Check sheet for the modelled part. Datum: model origin and axes. Units: mm. A direction names the side the tool comes from. Coordinates: 2 decimals unless noted, no trailing zeros. Write each loop counter-clockwise with the first axis right and the second up, starting at its lowest first coordinate (ties: lowest second). Pieces come first, ordered by that corner, then holes. Notation, with made-up numbers: (27, 75.5) -> (67, 75.5) arc R24 cw to (67, 87.5) -> close; hole circle Ø5 at (-37, -32). An arc over 180 degrees is marked (long way). Put each result on its own line as item: value.
```python
from build123d import *

# Parameters (mm, degrees)
SKETCH1_R           = 2.7
SKETCH1_R_2         = 3.55
BOSS_EXTRUDE1_DEPTH = 3.175
CHAMFER1_SIZE       = 3
CUT_EXTRUDE2_REACH  = 5.175
CUT_EXTRUDE3_START  = -3.175
SKETCH8_W           = 11
SKETCH8_H           = 1.8
CUT_EXTRUDE3_DEPTH  = 3.175
SKETCH9_W           = 8.878679656
SKETCH9_H           = 1.6
BOSS_EXTRUDE2_DEPTH = 3.175
BOSS_EXTRUDE3_DEPTH = 3.175
CUT_EXTRUDE4_REACH  = 5.175
CHAMFER3_SIZE       = 1.060660172
CHAMFER4_SIZE       = 3


with BuildPart() as part:
    # Sketch1 → Boss-Extrude1 (new body)
    with BuildSketch(Plane(origin=(0, 0, 0), x_dir=(1, 0, 0), z_dir=(0, 1, 0))):
        Polygon((0, 0), (40, 0), (40, -17.5), (57, -17.5), (57, 37.5), (40, 37.5), (40, 20), (0, 20), align=None)
        with Locations((29, 10)):
            Circle(SKETCH1_R, mode=Mode.SUBTRACT)
        with Locations((9, 10)):
            Circle(SKETCH1_R_2, mode=Mode.SUBTRACT)
        with Locations((48.5, 31.5)):
            Circle(SKETCH1_R, mode=Mode.SUBTRACT)
        with Locations((48.5, -11.5)):
            Circle(SKETCH1_R, mode=Mode.SUBTRACT)
        with Locations((49, 10)):
            Circle(SKETCH1_R, mode=Mode.SUBTRACT)
    extrude(amount=BOSS_EXTRUDE1_DEPTH)

    # Chamfer1
    chamfer1_edges = [part.edges().sort_by_distance(p)[0] for p in [
        (0, 1.5875, -20),
        (40, 1.5875, -37.5),
        (57, 1.5875, -37.5),
        (57, 1.5875, 17.5),
        (40, 1.5875, 17.5),
        (0, 1.5875, 0),
    ]]
    chamfer(chamfer1_edges, length=CHAMFER1_SIZE)

    # Sketch6 → Cut-Extrude2 (cut, up to next)
    with BuildSketch(Plane(origin=(0, 3.175, 0), x_dir=(1, 0, 0), z_dir=(0, 1, 0)), mode=Mode.PRIVATE) as cut_extrude2_sk1:
        Polygon((23.5, 16.560660172), (26.160660172, 13.9), (31.839339828, 13.9), (34.5, 16.560660172), (34.5, 18.2), (32.125, 18.2), (32.125, 18.545), (33.58, 20), (24.42, 20), (25.875, 18.545), (25.875, 18.2), (23.5, 18.2), align=None)
    cut_extrude2_tool1 = extrude(cut_extrude2_sk1.sketch, amount=-CUT_EXTRUDE2_REACH, mode=Mode.PRIVATE) & part.part
    add(cut_extrude2_tool1.solids().sort_by_distance((29, 3.175, -16.994051))[0], mode=Mode.SUBTRACT)

    # Sketch8 → Cut-Extrude3 (cut)
    with BuildSketch(Plane.XZ.offset(CUT_EXTRUDE3_START)):
        with Locations((29, -19.1)):
            Rectangle(SKETCH8_W, SKETCH8_H)
    extrude(amount=CUT_EXTRUDE3_DEPTH, mode=Mode.SUBTRACT)

    # Sketch9 → Boss-Extrude2 (add)
    with BuildSketch(Plane(origin=(0, 0, 0), x_dir=(-1, 0, 0), z_dir=(0, -1, 0))):
        with Locations((-29, 14.7)):
            Rectangle(SKETCH9_W, SKETCH9_H)
    extrude(amount=-BOSS_EXTRUDE2_DEPTH)

    # Sketch10 → Boss-Extrude3 (add)
    with BuildSketch(Plane.XZ):
        Polygon((40, -22.060660172), (40, -20), (37.939339828, -20), align=None)
    extrude(amount=-BOSS_EXTRUDE3_DEPTH)

    # Sketch11 → Cut-Extrude4 (cut, up to next)
    with BuildSketch(Plane.XZ, mode=Mode.PRIVATE) as cut_extrude4_sk1:
        Polygon((34.5, -16.560660172), (37.939339828, -20), (34.5, -20), align=None)
    cut_extrude4_tool1 = extrude(cut_extrude4_sk1.sketch, amount=-CUT_EXTRUDE4_REACH, mode=Mode.PRIVATE) & part.part
    add(cut_extrude4_tool1.solids().sort_by_distance((35.646447, 0, -18.853553))[0], mode=Mode.SUBTRACT)

    # Chamfer3
    chamfer3_edges = [part.edges().sort_by_distance(p)[0] for p in [
        (23.5, 1.5875, -20),
    ]]
    chamfer(chamfer3_edges, length=CHAMFER3_SIZE)

    # Chamfer4
    chamfer4_edges = [part.edges().sort_by_distance(p)[0] for p in [
        (40, 1.5875, 0),
    ]]
    chamfer(chamfer4_edges, length=CHAMFER4_SIZE)


solid = part.part
```
Q1. Cross-section at C-C (y = 1.4). Record the cut outline in (x, z).
Recorded:
outline: (0, -17) -> (3, -20) -> (22.44, -20) -> (23.5, -18.94) -> (23.5, -16.56) -> (24.56, -15.5) -> (33.44, -15.5) -> (40, -22.06) -> (40, -34.5) -> (43, -37.5) -> (54, -37.5) -> (57, -34.5) -> (57, 14.5) -> (54, 17.5) -> (43, 17.5) -> (40, 14.5) -> (40, 3) -> (37, 0) -> (3, 0) -> (0, -3) -> close; hole circle Ø7.1 at (9, -10); hole circle Ø5.4 at (29, -10); hole circle Ø5.4 at (48.5, -31.5); hole circle Ø5.4 at (48.5, 11.5); hole circle Ø5.4 at (49, -10)
Q2. Cross-section at B-B (x = 29). Record the cut outline in (y, z) (3 decimals), plus the area to 3 significant figures.
Recorded:
outline: (0, -15.5) -> (3.175, -15.5) -> (3.175, -12.7) -> (0, -12.7) -> close; (0, -7.3) -> (3.175, -7.3) -> (3.175, 0) -> (0, 0) -> close
area: 32.1 mm2
Q3. Depth check by flat-ended pin: P1, Ø1.6, axis at y = 1, z = -27.5, coming from the -X side; P2, Ø1.6, axis at x = 15, y = 2, coming from the +Z side; P3, Ø1, axis at x = 16, y = 1, coming from the -Z side. Enter the tip coordinate at first touch or a pass-through.
Recorded:
P1: stops at x = 40
P2: stops at z = 0
P3: stops at z = -20
Q4. Tool access check on faces 1 (the flat face through (29, 2, -15.5)), 2 (the flat face through (40, 2, 9)), 3 (the flat face through (13, 2, -20)), 4 (the flat face through (0, 2, -10)), 5 (the flat face through (34, 0, -10)). Record the directions out of +Z, -Z, +X, -X, +Y, -Y that give a thin tool (end or side, any length) a straight path to the whole face; none if there is none.
Recorded:
face 1: -Z, +Y, -Y
face 2: +Z, -X, +Y, -Y
face 3: -Z, -X, +Y, -Y
face 4: +Z, -Z, -X, +Y, -Y
face 5: +Z, -Z, +X, -X, -Y
Q5. Mould release check, pull along Z, two halves, no side actions. Record for faces 6 (the flat face through (41.5, 1.6, -36)), 7 (the flat face through (39, 2, 2)), 8 (the cylindrical face through (6.183, 1.565, -7.84)): released by +Z, released by -Z, zero draft, split by the parting line, or undercut.
Recorded:
face 6: released by -Z
face 7: released by +Z
face 8: undercut
Q6. Cross-section at A-A (z = -31.5). Record the cut outline in (x, y) (3 decimals).
Recorded:
outline: (40, 0) -> (45.8, 0) -> (45.8, 3.175) -> (40, 3.175) -> close; (51.2, 0) -> (57, 0) -> (57, 3.175) -> (51.2, 3.175) -> close
Q7. Cross-section at D-D (z = -10). Record the cut outline in (x, y) (3 decimals).
Recorded:
outline: (0, 0) -> (5.45, 0) -> (5.45, 3.175) -> (0, 3.175) -> close; (12.55, 0) -> (26.3, 0) -> (26.3, 3.175) -> (12.55, 3.175) -> close; (31.7, 0) -> (46.3, 0) -> (46.3, 3.175) -> (31.7, 3.175) -> close; (51.7, 0) -> (57, 0) -> (57, 3.175) -> (51.7, 3.175) -> close
Q8. Material ranges on line 1 along X through (y, z) = (2.3, -10); line 2 along Z through (x, y) = (29, 0.6); line 3 along X through (y, z) = (1.2, -31.5), recorded low to high.
Recorded:
line 1: x = 0 to 5.45, 12.55 to 26.3, 31.7 to 46.3, 51.7 to 57
line 2: z = -15.5 to -12.7, -7.3 to 0
line 3: x = 40 to 45.8, 51.2 to 57
